Verification items for the finished model (mm, model axes). A direction names the side the tool comes from. Coordinates: 2 decimals unless noted, no trailing zeros. Loops run counter-clockwise (first coordinate to the right, second up) from the corner with the lowest first, then second, coordinate; pieces in that order, holes last. Notation, with made-up numbers: (-5.75, 83.5) -> (29.25, 83.5) arc R24 cw to (29.25, 99.5) -> close; hole circle Ø9 at (22.25, 58). An arc over 180 degrees is marked (long way). Answer as a JSON object with one key per item and string values. Group by question number.
Q1. Gauge pin test, flat ends, axial feed: pin 1 Ø5.5 at (x, y) = (8.5, 9.5) entering from -Z; pin 2 Ø5 at (x, y) = (2.5, 5) entering from -Z. Record the tip position at first contact, or that the pin passes through.
Q2. Cross-section at D-D on z = 7.5. Record the boundary of the cut face in (x, y), and give its area (3 significant figures).
Q3. Set-up check for faces 4 (the flat face through (10, 19.655, 25)), 5 (the flat face through (19, 6, 19)): record each of +Z, -Z, +X, -X, +Y, -Y from which the full face is reachable in a straight line by a thin tool's end or side.
Q4. Cross-section at B-B on z = 19.75. Record the boundary of the cut face in (x, y), and give its area (3 significant figures).
Q5. Release check for a two-part mould opening along X. For faces 1 (the flat face through (19.49, 9.77, 16.14)), 2 (the flat face through (10, 11, 24.027)), 3 (the flat face through (0, 5, 20)) record: released by +X, released by -X, zero draft, split by the parting line, or undercut.
Q6. Scan lines: L1, parallel to X at y = 7, z = 22.75; L2, parallel to Z at x = 12.25, y = 10.5; L3, parallel to Y at x = 16.75, z = 16.25. Record each from-to range of solid material in increasing order.
Q7. Cross-section at A-A on y = 6.25. Record the boundary of the cut face in (x, z).
Q8. Cross-section at C-C on x = 6.25. Record the boundary of the cut face in (y, z).
```python
from build123d import *

# Parameters (mm, degrees)
EXTRUDE_1_DEPTH     = 20
CUT_EXTRUDE_START   = -2
SKETCH_3_W          = 18
SKETCH_3_H          = 16
CUT_EXTRUDE_1_DEPTH = 16


with BuildPart() as part:
    # 草图1 → 凸台-拉伸1 (new body)
    with BuildSketch(Plane(origin=(0, 0, 0), x_dir=(0, 0, -1), z_dir=(1, 0, 0))):
        Polygon((-6.026925143, -0.344583577), (-26.026925143, -0.344583577), (-26.026925143, 19.655416423), (-24.026925143, 19.655416423), (-24.026925143, 17.655416423), (-8.026925143, 1.655416423), (-6.026925143, 1.655416423), align=None)
    extrude(amount=EXTRUDE_1_DEPTH)

    # 草图3 → 切除-拉伸1 (cut)
    with BuildSketch(Plane.XZ.offset(0.344583577).offset(CUT_EXTRUDE_START)):
        with Locations((10, 16.026925143)):
            Rectangle(SKETCH_3_W, SKETCH_3_H)
    extrude(amount=-CUT_EXTRUDE_1_DEPTH, mode=Mode.SUBTRACT)


solid = part.part
```
Computed values:
{
 "1": {"pin 1": "stops at z = 24.03", "pin 2": "stops at z = 9.37"},
 "2": {"outline": "(0, -0.34) -> (20, -0.34) -> (20, 1.66) -> (0, 1.66) -> close", "area": "40.0 mm²"},
 "3": {"face 4": "+Z, -Z, +X, -X, +Y", "face 5": "-Z, +Y"},
 "4": {"outline": "(0, -0.34) -> (20, -0.34) -> (20, 13.38) -> (19, 13.38) -> (19, 1.66) -> (1, 1.66) -> (1, 13.38) -> (0, 13.38) -> close", "area": "63.4 mm²"},
 "5": {"face 1": "zero draft", "face 2": "undercut", "face 3": "released by -X"},
 "6": {"L1": "x = 0 to 1, 19 to 20", "L2": "z = 24.03 to 26.03", "L3": "y = -0.34 to 1.66"},
 "7": {"outline": "(0, 12.62) -> (1, 12.62) -> (1, 24.03) -> (19, 24.03) -> (19, 12.62) -> (20, 12.62) -> (20, 26.03) -> (0, 26.03) -> close"},
 "8": {"outline": "(-0.34, 6.03) -> (1.66, 6.03) -> (1.66, 24.03) -> (19.66, 24.03) -> (19.66, 26.03) -> (-0.34, 26.03) -> close"}
}
